For this review, take the finished solid that the model builds, in its own axes (mm). Round coordinates to 2 decimals unless told otherwise and drop trailing zeros. Write each loop counter-clockwise with the first axis right and the second up, starting at its lowest first coordinate (ties: lowest second). Pieces come first, ordered by that corner, then holes. Notation, with made-up numbers: (-35.75, -20) - (14.25, -20) arc R25 cw to (14.25, 14) - close; hole circle Ø8 at (80.25, 83.5). An arc over 180 degrees is marked (long way). One line per item, written item: value. Start each with the question number.
Q1. For probe 1 along X at (y, z) = (1.6, -166), list the stretches that pass through material, from the lowest coordinate up.
Q2. Clearance check with flat-ended pins moving along their axes: pin 1 Ø10 at (x, z) = (1291.5, 37) entering from -Y; pin 2 Ø0.6 at (x, y) = (421.5, 1) entering from -Z; pin 3 Ø1 at (x, y) = (1193.5, 1.5) entering from +Z; pin 4 Ø0.6 at (y, z) = (0.5, 66) entering from +X. State where each tip first meets the part, or that it passes through.
Q3. Add section A-A on z = -220. Write out the cut boundary in (x, y).
```python
from build123d import *

# Parameters (mm, degrees)
BOSS_EXTRUDE1_DEPTH = 2


with BuildPart() as part:
    # Sketch1 → Boss-Extrude1 (new body)
    with BuildSketch(Plane(origin=(0, 0, 0), x_dir=(1, 0, 0), z_dir=(0, 1, 0))):
        Polygon((0, 0), (0, 296), (416, 296), (416, 119), (426, 119), (426, 296), (766, 296), (766, 119), (776, 119), (776, 296), (1189, 296), (1189, 119), (1199, 119), (1199, 296), (1539, 296), (1539, 119), (1544, 119), (1582, 112.299574733), (1582, 6.700425267), (1544, 0), (1539, 0), (1539, -177), (1199, -177), (1199, 0), (1189, 0), (1189, -177), (776, -177), (776, 0), (766, 0), (766, -177), (426, -177), (426, 0), (416, 0), (416, -177), (0, -177), align=None)
    extrude(amount=BOSS_EXTRUDE1_DEPTH)


solid = part.part
```
Result set:
1. probe 1: x = 0 to 416, 426 to 766, 776 to 1189, 1199 to 1539
2. pin 1: stops at y = 0
2. pin 2: stops at z = -119
2. pin 3: stops at z = 0
2. pin 4: stops at x = 1539
3. outline: (0, 0) - (416, 0) - (416, 2) - (0, 2) - close; (426, 0) - (766, 0) - (766, 2) - (426, 2) - close; (776, 0) - (1189, 0) - (1189, 2) - (776, 2) - close; (1199, 0) - (1539, 0) - (1539, 2) - (1199, 2) - close
